```python
from build123d import *

# Parameters (mm, degrees)
F0_R     = 3.937
F0_R_2   = 2.667
F1_DEPTH = 2.794
F2_R     = 5.08
F3_DEPTH = 1.9812
F4_R     = 11.049
F5_DEPTH = 1.524


# Not quite as in the source:
# - a feature names something its author has since deleted; it is built from what else it names


with BuildPart() as f1:
    # F0 (on Top) → F1 (new body)
    with BuildSketch(Plane.XY):
        Circle(F0_R)
        Circle(F0_R_2, mode=Mode.SUBTRACT)
    extrude(amount=F1_DEPTH)

    # F2 (on face) → F3 (join)
    with BuildSketch(Plane(origin=(0, 0, 0), x_dir=(1, 0, 0), z_dir=(0, 0, -1))):
        Circle(F2_R)
    extrude(amount=F3_DEPTH)

    # F4 (on face) → F5 (join)
    with BuildSketch(Plane(origin=(0, 0, -1.9812), x_dir=(1, 0, 0), z_dir=(0, 0, -1))):
        Circle(F4_R)
    extrude(amount=F5_DEPTH)

    # F6 (on Front) → F7 (revolve)
    with BuildSketch(Plane.XZ):
        with BuildLine():
            Line((0, -2.54), (-11.09184091, -2.54))
            ThreePointArc((-11.09184091, -2.54), (-7.8431159233, -10.3831159233), (0, -13.63184091))
            Line((0, -13.63184091), (0, -3.5557490773))
            Line((0, -3.5557490773), (0, -2.54))
        make_face()
    revolve(axis=Axis((0, 0, -8.5937949937), (0, 0, -1)))


solid = f1.part
```
Build history of the part. All positions in model axes, mm. A direction names the side the tool comes from. Round coordinates to 2 decimals unless told otherwise and drop trailing zeros. Order: outer loops, then holes, each group sorted by start corner. A loop starts at its lowest first (then second) coordinate and runs counter-clockwise, first axis right, second up. Notation, with made-up numbers: (-36, 3) - (-27, 3) arc R27 cw to (-27, 39) - close; hole circle Ø5 at (62.25, -11.5). An arc over 180 degrees is marked (long way). Use a Markdown table: item, result.
1) Tool access for faces 1 (the face through (3, -1, 2.794)), 2 (the face through (-1.438, -10.955, -2.257)): list every direction of +Z, -Z, +X, -X, +Y, -Y with a clear straight run to the whole face (end or side of a thin tool).
Recorded:
| item | result |
|---|---|
| face 1 | +Z, +X, -X, +Y, -Y |
| face 2 | +Z |
2) Saw through at C-C on z = -0.5. Write the cut outline in (x, y).
Recorded:
| item | result |
|---|---|
| outline | circle Ø10.16 at (0, 0) |
3) Saw through at D-D on x = -4.25. Write the cut outline in (y, z), and give its area (3 significant figures).
Recorded:
| item | result |
|---|---|
| outline | (-10.25, -2.54) arc R10.25 ccw to (10.25, -2.54) - (10.2, -2.54) - (10.2, -1.98) - (2.78, -1.98) - (2.78, 0) - (-2.78, 0) - (-2.78, -1.98) - (-10.2, -1.98) - (-10.2, -2.54) - close |
| area | 187 mm² |
4) Saw through at A-A on y = 0. Write the cut outline in (x, z).
Recorded:
| item | result |
|---|---|
| outline | (-11.09, -2.54) arc R11.09 ccw to (11.09, -2.54) - (11.05, -2.54) - (11.05, -1.98) - (5.08, -1.98) - (5.08, 0) - (3.94, 0) - (3.94, 2.79) - (2.67, 2.79) - (2.67, 0) - (-2.67, 0) - (-2.67, 2.79) - (-3.94, 2.79) - (-3.94, 0) - (-5.08, 0) - (-5.08, -1.98) - (-11.05, -1.98) - (-11.05, -2.54) - close |
5) Flat gauge pins, fed straight in: pin 1 Ø1 at (x, z) = (-1, -4) entering from +Y; pin 2 Ø1 at (y, z) = (0.5, -6.5) entering from +X; pin 3 Ø8 at (x, z) = (1, -9) entering from -Y; pin 4 Ø6 at (x, y) = (0, 0) entering from +Z. Where does each tip first touch, or does it go through?
Recorded:
| item | result |
|---|---|
| pin 1 | stops at y = 11.02 |
| pin 2 | stops at x = 10.53 |
| pin 3 | stops at y = -10.8 |
| pin 4 | stops at z = 2.79 |
6) Wall check: L1, parallel to Y at x = 0, z = 0.8; L2, parallel to Y at x = -1.25, z = -8; L3, parallel to Y at x = -4, z = -6. Give the ranges that are in metal, low to high.
Recorded:
| item | result |
|---|---|
| L1 | y = -3.94 to -2.67, 2.67 to 3.94 |
| L2 | y = -9.57 to 9.57 |
| L3 | y = -9.75 to 9.75 |
7) Pull direction Y, two halves, no side cores. Call faces 3 (the face through (0, 0, 0)), 4 (the face through (5, 2, -1.981)), 5 (the face through (-0.661, -5.037, -0.977)): pulls with the +Y half, pulls with the -Y half, needs draft (parallel to the pull), parting line crosses it, or undercut.
Recorded:
| item | result |
|---|---|
| face 3 | undercut |
| face 4 | needs draft |
| face 5 | parting line crosses it |
